Autodesk Fusion 360 part; units mm, degrees
sketch "Sketch1" plane through (0, 0, 0) normal (0, 0, 1) x (1, 0, 0)
  line L0 (0, 0) -> (262, 0)
  line L1 (262, 0) -> (262, 100.0014)
  line L2 (262, 100.0014) -> (0, 100.0014)
  line L3 (0, 100.0014) -> (0, 0)
extrude "Extrude1" add sketch "Sketch1" along normal blind 3
sketch "Sketch2" plane through (0, 0, 3) normal (0, 0, 1) x (-1, 0, 0)
  line L0 (0, -100.0014) -> (0, 0)
  line L1 (0, 0) -> (-262, 0)
  line L2 (-262, 0) -> (-262, -100.0014)
  line L3 (-262, -100.0014) -> (0, -100.0014)
  line L4 (-141.5, -69) -> (-141.5, -84)
  line L5 (-188.5, -84) -> (-188.5, -69)
  line L6 (-141.5, -84) -> (-188.5, -84)
  line L7 (-188.5, -69) -> (-141.5, -69)
  line L8 (-216.5, -84) -> (-248.5, -84)
  line L9 (-216.5, -69) -> (-216.5, -84)
  line L10 (-248.5, -69) -> (-216.5, -69)
  line L11 (-248.5, -84) -> (-248.5, -69)
  line L12 (-16.5, -84) -> (-48.5, -84)
  line L13 (-48.5, -84) -> (-48.5, -69)
  line L14 (-16.5, -69) -> (-16.5, -84)
  line L15 (-48.5, -69) -> (-16.5, -69)
  line L16 (-98.5, -69) -> (-66.5, -69)
  line L17 (-98.5, -84) -> (-98.5, -69)
  line L18 (-66.5, -84) -> (-98.5, -84)
  line L19 (-66.5, -69) -> (-66.5, -84)
  line L20 (-113, -25) -> (-130.6, -25)
  line L21 (-130.6, -25) -> (-130.6, -7.4)
  line L22 (-130.6, -7.4) -> (-113, -7.4)
  line L23 (-113, -7.4) -> (-113, -25)
  line L24 (-144.6, -53) -> (-144.6, -35.4)
  line L25 (-127, -53) -> (-144.6, -53)
  line L26 (-127, -35.4) -> (-127, -53)
  line L27 (-144.6, -35.4) -> (-127, -35.4)
  line L28 (-116.6, -53) -> (-116.6, -35.4)
  line L29 (-99, -53) -> (-116.6, -53)
  line L30 (-99, -35.4) -> (-99, -53)
  line L31 (-116.6, -35.4) -> (-99, -35.4)
  circle A0 centre (-35, -43) radius 3.8
  circle A1 centre (-79, -43) radius 3.8
  circle A2 centre (-170, -43) radius 3.8
  circle A3 centre (-230, -43) radius 3.8
  circle A4 centre (-122, -64) radius 4
  circle A5 centre (-14, -55) radius 4
  circle A6 centre (-204, -58) radius 4
  line L32 (-87.6, -25) -> (-87.6, -7.4)
  line L33 (-70, -25) -> (-87.6, -25)
  line L34 (-70, -7.4) -> (-70, -25)
  line L35 (-87.6, -7.4) -> (-70, -7.4)
  line L36 (-178.6, -25) -> (-178.6, -7.4)
  line L37 (-161, -25) -> (-178.6, -25)
  line L38 (-161, -7.4) -> (-161, -25)
  line L39 (-178.6, -7.4) -> (-161, -7.4)
  line L40 (-238.6, -25) -> (-238.6, -7.4)
  line L41 (-221, -25) -> (-238.6, -25)
  line L42 (-221, -7.4) -> (-221, -25)
  line L43 (-238.6, -7.4) -> (-221, -7.4)
  point P0 (-56, -93.0014)
  dimension "d15" = 47
  dimension "d16" = 15
  dimension "d17" = 32
  dimension "d18" = 15
  dimension "d19" = 32
  dimension "d20" = 15
  dimension "d21" = 32
  dimension "d22" = 15
  dimension "d24" = 17.6
  dimension "d25" = 17.6
  dimension "d26" = 17.6
  dimension "d27" = 17.6
  dimension "d28" = 17.6
  dimension "d29" = 17.6
  dimension "d31" = 7.6
  dimension "d32" = 7.6
  dimension "d33" = 7.6
  dimension "d34" = 7.6
  dimension "d35" = 8
  dimension "d36" = 8
  dimension "d37" = 8
  dimension "d38" = 17.6
  dimension "d39" = 17.6
  dimension "d40" = 17.6
  dimension "d41" = 17.6
  dimension "d42" = 17.6
  dimension "d43" = 17.6
extrude "Extrude2" cut sketch "Sketch2" against normal blind 20 contours L4 L5 L6 L7 | L8 L9 L10 L11 | L12 L13 L14 L15 | L16 L17 L18 L19 | L20 L21 L22 L23 | L24 L25 L26 L27 | L28 L29 L30 L31 | A0 | A1 | A2 | A3 | A4 | A5 | A6 | L32 L33 L34 L35 | L36 L37 L38 L39 | L40 L41 L42 L43
sketch "Sketch3" plane through (0, 0, 0) normal (0, 0, -1) x (1, 0, 0)
  circle A0 centre (170, -43) radius 3.8
  line L0 (216.5, -84) -> (216.5, -69)
  line L1 (216.5, -69) -> (248.5, -69)
  line L2 (248.5, -69) -> (248.5, -84)
  line L3 (248.5, -84) -> (216.5, -84)
  line L4 (130.6, -7.4) -> (130.6, -25)
  line L5 (130.6, -25) -> (113, -25)
  line L6 (113, -25) -> (113, -7.4)
  line L7 (113, -7.4) -> (130.6, -7.4)
  line L8 (98.5, -69) -> (98.5, -84)
  line L9 (98.5, -84) -> (66.5, -84)
  line L10 (66.5, -84) -> (66.5, -69)
  line L11 (66.5, -69) -> (98.5, -69)
  line L12 (116.6, -53) -> (99, -53)
  line L13 (99, -53) -> (99, -35.4)
  line L14 (99, -35.4) -> (116.6, -35.4)
  line L15 (116.6, -35.4) -> (116.6, -53)
  line L16 (87.6, -25) -> (70, -25)
  line L17 (70, -25) -> (70, -7.4)
  line L18 (70, -7.4) -> (87.6, -7.4)
  line L19 (87.6, -7.4) -> (87.6, -25)
  line L20 (188.5, -84) -> (141.5, -84)
  line L21 (141.5, -84) -> (141.5, -69)
  line L22 (141.5, -69) -> (188.5, -69)
  line L23 (188.5, -69) -> (188.5, -84)
  circle A1 centre (204, -58) radius 4
  circle A2 centre (35, -43) radius 3.8
  line L24 (238.6, -25) -> (221, -25)
  line L25 (221, -25) -> (221, -7.4)
  line L26 (221, -7.4) -> (238.6, -7.4)
  line L27 (238.6, -7.4) -> (238.6, -25)
  line L28 (144.6, -53) -> (127, -53)
  line L29 (127, -53) -> (127, -35.4)
  line L30 (127, -35.4) -> (144.6, -35.4)
  line L31 (144.6, -35.4) -> (144.6, -53)
  circle A3 centre (79, -43) radius 3.8
  circle A4 centre (122, -64) radius 4
  line L32 (48.5, -84) -> (16.5, -84)
  line L33 (16.5, -84) -> (16.5, -69)
  line L34 (16.5, -69) -> (48.5, -69)
  line L35 (48.5, -69) -> (48.5, -84)
  line L36 (178.6, -25) -> (161, -25)
  line L37 (161, -25) -> (161, -7.4)
  line L38 (161, -7.4) -> (178.6, -7.4)
  line L39 (178.6, -7.4) -> (178.6, -25)
  circle A5 centre (230, -43) radius 3.8
  circle A6 centre (14, -55) radius 4
  line L40 (0, 0) -> (0, -100.0014)
  line L41 (0, -100.0014) -> (262, -100.0014)
  line L42 (262, -100.0014) -> (262, 0)
  line L43 (262, 0) -> (0, 0)
  circle A7 centre (6.5, -6.5) radius 0.85
  dimension "d46" = 1.7
extrude "Extrude3" cut sketch "Sketch3" against normal blind 4 contours A7
sketch "Sketch4" plane through (0, 0, 0) normal (0, 0, -1) x (1, 0, 0)
  circle A0 centre (6.5, -6.5) radius 0.85
  circle A1 centre (170, -43) radius 3.8
  line L0 (216.5, -84) -> (216.5, -69)
  line L1 (216.5, -69) -> (248.5, -69)
  line L2 (248.5, -69) -> (248.5, -84)
  line L3 (248.5, -84) -> (216.5, -84)
  line L4 (130.6, -7.4) -> (130.6, -25)
  line L5 (130.6, -25) -> (113, -25)
  line L6 (113, -25) -> (113, -7.4)
  line L7 (113, -7.4) -> (130.6, -7.4)
  line L8 (98.5, -69) -> (98.5, -84)
  line L9 (98.5, -84) -> (66.5, -84)
  line L10 (66.5, -84) -> (66.5, -69)
  line L11 (66.5, -69) -> (98.5, -69)
  line L12 (116.6, -53) -> (99, -53)
  line L13 (99, -53) -> (99, -35.4)
  line L14 (99, -35.4) -> (116.6, -35.4)
  line L15 (116.6, -35.4) -> (116.6, -53)
  line L16 (87.6, -25) -> (70, -25)
  line L17 (70, -25) -> (70, -7.4)
  line L18 (70, -7.4) -> (87.6, -7.4)
  line L19 (87.6, -7.4) -> (87.6, -25)
  line L20 (188.5, -84) -> (141.5, -84)
  line L21 (141.5, -84) -> (141.5, -69)
  line L22 (141.5, -69) -> (188.5, -69)
  line L23 (188.5, -69) -> (188.5, -84)
  circle A2 centre (204, -58) radius 4
  circle A3 centre (35, -43) radius 3.8
  line L24 (238.6, -25) -> (221, -25)
  line L25 (221, -25) -> (221, -7.4)
  line L26 (221, -7.4) -> (238.6, -7.4)
  line L27 (238.6, -7.4) -> (238.6, -25)
  line L28 (144.6, -53) -> (127, -53)
  line L29 (127, -53) -> (127, -35.4)
  line L30 (127, -35.4) -> (144.6, -35.4)
  line L31 (144.6, -35.4) -> (144.6, -53)
  circle A4 centre (79, -43) radius 3.8
  circle A5 centre (122, -64) radius 4
  line L32 (48.5, -84) -> (16.5, -84)
  line L33 (16.5, -84) -> (16.5, -69)
  line L34 (16.5, -69) -> (48.5, -69)
  line L35 (48.5, -69) -> (48.5, -84)
  line L36 (178.6, -25) -> (161, -25)
  line L37 (161, -25) -> (161, -7.4)
  line L38 (161, -7.4) -> (178.6, -7.4)
  line L39 (178.6, -7.4) -> (178.6, -25)
  circle A6 centre (230, -43) radius 3.8
  circle A7 centre (14, -55) radius 4
  line L40 (0, 0) -> (0, -100.0014)
  line L41 (0, -100.0014) -> (262, -100.0014)
  line L42 (262, -100.0014) -> (262, 0)
  line L43 (262, 0) -> (0, 0)
  circle A8 centre (255.2, -93.2014) radius 0.85
  dimension "d49" = 1.7
extrude "Extrude4" cut sketch "Sketch4" against normal blind 5 contours A8
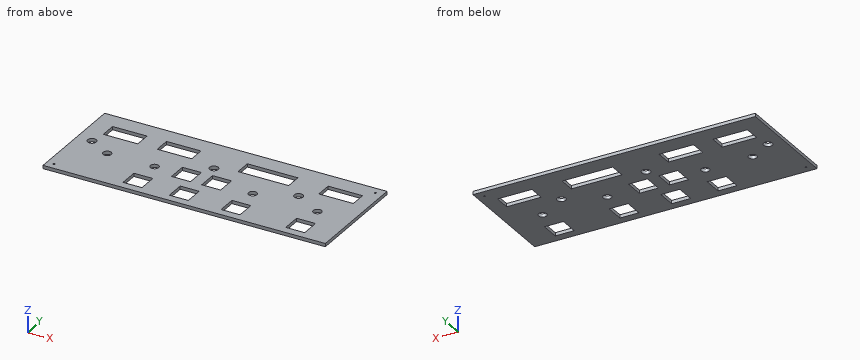
Geometry check sheet. Reference: the model listing, model coordinates, mm. Coordinates: 2 decimals unless noted, no trailing zeros. Order: outer loops, then holes, each group sorted by start corner. A loop starts at its lowest first (then second) coordinate and runs counter-clockwise, first axis right, second up.
Q1. Thickness scan on probe 1 along X at (y, z) = (74.5, 0.35); probe 2 along Y at (x, z) = (163, 0.25); probe 3 along X at (y, z) = (35.5, 2.1). Record the ranges inside material, lowest first.
Reply:
probe 1: x = 0 to 16.5, 48.5 to 66.5, 98.5 to 141.5, 188.5 to 216.5, 248.5 to 262
probe 2: y = 0 to 7.4, 25 to 69, 84 to 100
probe 3: x = 0 to 99, 116.6 to 127, 144.6 to 262
Q2. Sectioned sample at C-C on x = 170. Record the cut outline in (y, z).
Reply:
outline: (0, 0) - (7.4, 0) - (7.4, 3) - (0, 3) - close; (25, 0) - (39.2, 0) - (39.2, 3) - (25, 3) - close; (46.8, 0) - (69, 0) - (69, 3) - (46.8, 3) - close; (84, 0) - (100, 0) - (100, 3) - (84, 3) - close
Q3. Sectioned sample at B-B on y = 43. Record the cut outline in (x, z), and give its area (3 significant figures).
Reply:
outline: (0, 0) - (31.2, 0) - (31.2, 3) - (0, 3) - close; (38.8, 0) - (75.2, 0) - (75.2, 3) - (38.8, 3) - close; (82.8, 0) - (99, 0) - (99, 3) - (82.8, 3) - close; (116.6, 0) - (127, 0) - (127, 3) - (116.6, 3) - close; (144.6, 0) - (166.2, 0) - (166.2, 3) - (144.6, 3) - close; (173.8, 0) - (226.2, 0) - (226.2, 3) - (173.8, 3) - close; (233.8, 0) - (262, 0) - (262, 3) - (233.8, 3) - close
area: 589 mm2
Q4. Sectioned sample at A-A on x = 35. Record the cut outline in (y, z), and give its area (3 significant figures).
Reply:
outline: (0, 0) - (39.2, 0) - (39.2, 3) - (0, 3) - close; (46.8, 0) - (69, 0) - (69, 3) - (46.8, 3) - close; (84, 0) - (100, 0) - (100, 3) - (84, 3) - close
area: 232 mm2
Q5. Sectioned sample at D-D on x = 122. Record the cut outline in (y, z).
Reply:
outline: (0, 0) - (7.4, 0) - (7.4, 3) - (0, 3) - close; (25, 0) - (60, 0) - (60, 3) - (25, 3) - close; (68, 0) - (100, 0) - (100, 3) - (68, 3) - close
